```python
from build123d import *

# Parameters (mm, degrees)
F1_DEPTH  = 426
F3_DEPTH  = 4
F4_R      = 2
F7_DEPTH  = 4
F10_DEPTH = 4


# Not quite as in the source:
# - a feature names something its author has since deleted; it is built from what else it names


with BuildPart() as f1:
    # F0 (on Top) → F1 (new body)
    with BuildSketch(Plane.XY):
        Polygon((-200, -343), (0, -343), (0, 0), (-495, 0), (-495, -1261), (-492.1838745495, -1261), (-492.1838745495, -4), (-4, -4), (-4, -339), (-204, -339), (-204, -1261), (-200, -1261), align=None)
    extrude(amount=F1_DEPTH)

    # F2 (on Top) → F3 (join)
    with BuildSketch(Plane.XY):
        Polygon((0, 0), (-495, 0), (-495, -1261), (-200, -1261), (-200, -343), (0, -343), align=None)
    extrude(amount=-F3_DEPTH)

    # F4
    f4_edges = [f1.edges().sort_by_distance(p)[0] for p in [
        (-200, -802, -4),
        (-495, -630.5, -4),
        (-247.5, 0, -4),
        (0, -343, 211),
        (0, 0, 211),
    ]]
    fillet(f4_edges, radius=F4_R)

    # F6 (on offset) → F7 (join)
    with BuildSketch(Plane.XZ.offset(961)):
        Polygon((-492.1838745495, 355), (-492.1838745495, 0), (-270.1838745495, 0), align=None)
    extrude(amount=F7_DEPTH)

    # F9 (on offset) → F10 (join)
    with BuildSketch(Plane.XZ.offset(361)):
        Polygon((-204, 355), (-426, 0), (-204, 0), align=None)
    extrude(amount=F10_DEPTH)


solid = f1.part
```
Check sheet for the modelled part. Datum: model origin and axes. Units: mm. A direction names the side the tool comes from. Round coordinates to 2 decimals unless told otherwise and drop trailing zeros. Order: outer loops, then holes, each group sorted by start corner. A loop starts at its lowest first (then second) coordinate and runs counter-clockwise, first axis right, second up. Notation, with made-up numbers: (81, -23.5) - (112, -23.5) arc R28 cw to (112, -1.5) - close; hole circle Ø10 at (-10.75, 25.5). An arc over 180 degrees is marked (long way). Answer as CSV lines item,"result". Start each with the question number.
1) Depth check by flat-ended pin: pin 1 (12 mm diameter, centred on x = -86, z = 201, fed in from -Y); pin 2 (2 mm diameter, centred on y = -890, z = 230.5, fed in from +X); pin 3 (4 mm diameter, centred on x = -284.5, z = 231.5, fed in from -Y). Enter the tip coordinate at first touch or a pass-through.
2) Section check A-A (y = -610). Record the cut outline in (x, z).
3) Draft check along X on faces 1 (the face through (-204, -794, 210)), 2 (the face through (-103, -343, 214)), 3 (the face through (-495, -622, 215)). Enter one of: +X half, -X half, draft (parallel to the pull), parting line (faces both ways), or undercut.
4) Section check C-C (z = 187). Record the cut outline in (x, y), then the cut area to 3 significant figures.
5) Section check D-D (y = -81.5). Record the cut outline in (x, z).
6) Scan lines: probe 1 along Y at (x, z) = (-179, 207); probe 2 along X at (y, z) = (-1173, 75); probe 3 along X at (y, z) = (-59, 270). Record each from-to range of solid material in increasing order.
7) Section check B-B (x = -127). Record the cut outline in (y, z).
8) Tool access check on faces 4 (the face through (-432, -965, 101)), 5 (the face through (0, -174, 214)), 6 (the face through (-200, -808, 215)), 7 (the face through (-245, 0, 215)), 8 (the face through (-313.45, -362.97, 179.98)). Record the directions out of +Z, -Z, +X, -X, +Y, -Y that give a thin tool (end or side, any length) a straight path to the whole face; none if there is none.
Determined:
1,pin 1,"y = -343"
1,pin 2,"x = -200"
1,pin 3,"y = -4"
2,outline,"(-495, -2) arc R2 ccw to (-493, -4) - (-202, -4) arc R2 ccw to (-200, -2) - (-200, 426) - (-204, 426) - (-204, 0) - (-492.18, 0) - (-492.18, 426) - (-495, 426) - close"
3,face 1,"undercut"
3,face 2,"draft"
3,face 3,"-X half"
4,outline,"(-495, -1261) - (-492.18, -1261) - (-492.18, -965) - (-387.12, -965) - (-387.12, -961) - (-492.18, -961) - (-492.18, -4) - (-4, -4) - (-4, -339) - (-204, -339) - (-204, -361) - (-309.06, -361) - (-309.06, -365) - (-204, -365) - (-204, -1261) - (-200, -1261) - (-200, -343) - (-2, -343) arc R2 ccw to (0, -341) - (0, -2) arc R2 ccw to (-2, 0) - (-495, 0) - close"
4,area,"12,200 mm^2"
5,outline,"(-495, -2) arc R2 ccw to (-493, -4) - (0, -4) - (0, 426) - (-4, 426) - (-4, 0) - (-492.18, 0) - (-492.18, 426) - (-495, 426) - close"
6,probe 1,"-343 to -339, -4 to 0"
6,probe 2,"-495 to -492.18, -204 to -200"
6,probe 3,"-495 to -492.18, -4 to 0"
7,outline,"(-343, -4) - (-2, -4) arc R2 ccw to (0, -2) - (0, 426) - (-4, 426) - (-4, 0) - (-339, 0) - (-339, 426) - (-343, 426) - close"
8,face 4,"+Z, -Y"
8,face 5,"+Z, -Z, +X, +Y, -Y"
8,face 6,"+Z, -Z, +X, -Y"
8,face 7,"+Z, -Z, +X, -X, +Y"
8,face 8,"+Z"
